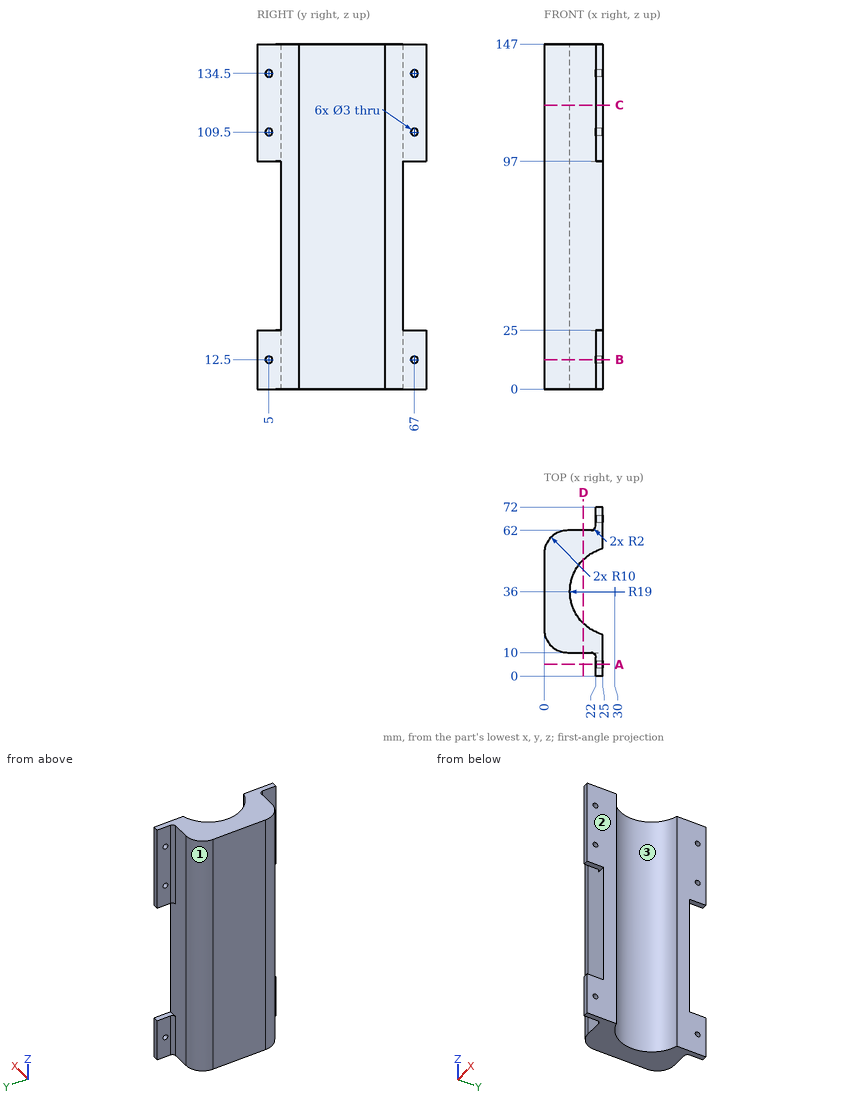
Input: dimensioned drawing with shaded views. Units: mm. Origin: part minimum x, y, z. Give positions to 0.01 mm unless a question says otherwise; leave off trailing zeros. Write each loop counter-clockwise with the first axis right and the second up, starting at its lowest first coordinate (ties: lowest second). Pieces come first, ordered by that corner, then holes. Notation, with made-up numbers: M 79.25,39 L 105.25,39 A19 ccw 105.25,70 Z; hole C 27.25,76 d3. An arc over 180 degrees is marked long. Write item = value, one per line. Start each with the question number.
1) Cut plane B-B on z = 12.5. Return the cut outline in (x, y), then the cut area to 3 significant figures.
2) Cut plane C-C on z = 121. Return the cut outline in (x, y).
3) First-contact query: pin 1 Ø6.5 at (y, z) = (4, 6.5) entering from -X; pin 2 Ø3 at (x, z) = (22, 41) entering from -Y; pin 3 Ø1 at (x, z) = (22, 67.5) entering from +Y. Flat tips, straight axial feed; report the tip coordinate or a pass-through.
4) Draft query along Y for the marked faces 1, 2 and 3. Return one class per face: +Y half, -Y half, draft (parallel to the pull), parting line (faces both ways), or undercut.
5) Cut plane A-A on y = 5. Return the cut outline in (x, z), then the cut area to 3 significant figures.
6) Material intervals for line 1 along Y through (x, z) = (24.15, 109.5); line 2 along Y through (x, z) = (9.5, 90); line 3 along X through (y, z) = (5, 20.5), sorted ascending. Write a range as [from, to].
7) Cut plane D-D on x = 16.75. Return the cut outline in (y, z).
Solved:
q1.outline = M 0,20 A10 ccw 10,10 L 20,10 A2 cw 22,8 L 22,6.5 L 25,6.5 L 25,17.67 A19 cw 25,54.33 L 25,65.5 L 22,65.5 L 22,64 A2 cw 20,62 L 10,62 A10 ccw 0,52 Z; M 22,0 L 25,0 L 25,3.5 L 22,3.5 Z; M 22,68.5 L 25,68.5 L 25,72 L 22,72 Z
q1.area = 922 mm2
q2.outline = M 0,20 A10 ccw 10,10 L 20,10 A2 cw 22,8 L 22,0 L 25,0 L 25,17.67 A19 cw 25,54.33 L 25,72 L 22,72 L 22,64 A2 cw 20,62 L 10,62 A10 ccw 0,52 Z
q3.pin_1 = 22
q3.pin_2 = 10
q3.pin_3 = 62
q4.face_1 = +Y half
q4.face_2 = draft
q4.face_3 = undercut
q5.outline = M 22,0 L 25,0 L 25,11 L 22,11 Z; M 22,14 L 25,14 L 25,25 L 22,25 Z; M 22,97 L 25,97 L 25,108 L 22,108 Z; M 22,111 L 25,111 L 25,133 L 22,133 Z; M 22,136 L 25,136 L 25,147 L 22,147 Z
q5.area = 198 mm2
q6.line_1 = [0, 3.5], [6.5, 17.92], [54.08, 65.5], [68.5, 72]
q6.line_2 = [10.01, 61.99]
q6.line_3 = [22, 25]
q7.outline = M 10,0 L 22.38,0 L 22.38,147 L 10,147 Z; M 49.62,0 L 62,0 L 62,147 L 49.62,147 Z
